```python
from build123d import *

# Parameters (mm, degrees)
F2_R     = 4.5
F3_DEPTH = 8
F4_W     = 30
F4_H     = 2
F5_DEPTH = 4.4


with BuildPart() as f1:
    # F0 (on Front) → F1 (revolve)
    with BuildSketch(Plane.XZ):
        Polygon((-7, 0), (0, 0), (0, 10), (-5, 10), (-5.25, 5.6), (-5, 5.6), (-5, 2), (-7, 2), align=None)
    revolve(axis=Axis((0, 0, 5), (0, 0, -1)))

    # F2 (on face) → F3 (cut)
    with BuildSketch(Plane.XY.offset(10)):
        Circle(F2_R)
    extrude(amount=-F3_DEPTH, mode=Mode.SUBTRACT)

    # F4 (on face) → F5 (cut)
    with BuildSketch(Plane.XY.offset(10)):
        with Locations((0.8593, 0)):
            Rectangle(F4_W, F4_H)
        with BuildLine():
            Line((-4.387482, 1), (4.387482, 1))
            ThreePointArc((4.387482, 1), (0, 4.5), (-4.387482, 1))
        make_face()
        with BuildLine():
            Line((15.8593, -1), (15.8593, 1))
            Line((15.8593, 1), (4.387482, 1))
            ThreePointArc((4.387482, 1), (4.471782, 0.503155), (4.5, 0))
            ThreePointArc((4.5, 0), (4.471782, -0.503155), (4.387482, -1))
            Line((4.387482, -1), (15.8593, -1))
        make_face()
    extrude(amount=-F5_DEPTH, mode=Mode.SUBTRACT)


solid = f1.part
```
Model file for the job. Use its own axes, mm. A direction names the side the tool comes from. Coordinates: 2 decimals unless noted, no trailing zeros. Loops run counter-clockwise (first coordinate to the right, second up) from the corner with the lowest first, then second, coordinate; pieces in that order, holes last. Notation, with made-up numbers: M -22,34.5 L -7,34.5 A16 ccw -7,63.5 Z; hole C -3,-40 d1. An arc over 180 degrees is marked long. Use CSV: the item, a comma, the result in double quotes. Start each with the question number.
1. Band-saw the part on D-D, the plane z = 4. List the corners of the cut face in (x, y), then the cut area to 3 significant figures.
2. Band-saw the part on B-B, the plane z = 7.75. List the corners of the cut face in (x, y).
3. Probe probe 1 along X at (y, z) = (0, 5.5); probe 2 along Y at (x, z) = (-3.25, 7.75). List the from-to ranges inside material, lowest first. Write a range as [from, to].
4. Band-saw the part on C-C, the plane y = 0. List the corners of the cut face in (x, z).
5. Two-plate mould, pull along Z, no slides. Class faces 1 (the cylindrical face through (-6.466, -2.681, 0.986)), 2 (the cylindrical face through (1.08, -4.88, 3.77)), 3 (the conical face through (-0.099, 5.126, 7.769)): pulls with the +Z half, pulls with the -Z half, needs draft (parallel to the pull), parting line crosses it, or undercut.
6. Tool access for faces 4 (the flat face through (0, 0, 2)), 5 (the conical face through (0.099, -5.126, 7.769)): list every direction of +Z, -Z, +X, -X, +Y, -Y with a clear straight run to the whole face (end or side of a thin tool).
7. Flat gauge pins, fed straight in: pin 1 (0.7 mm diameter, centred on x = -4.5, y = -0.5, fed in from +Z); pin 2 (0.8 mm diameter, centred on x = -4.5, z = 7, fed in from -Y); pin 3 (1.5 mm diameter, centred on x = -3, y = 5.5, fed in from +Z). Where does each tip first touch, or does it go through?
8. Band-saw the part on A-A, the plane x = 0. List the corners of the cut face in (y, z).
Entries:
1,outline,"C 0,0 d10; hole C 0,0 d9"
1,area,"14.9 mm2"
2,outline,"M -5.03,-1 A5.13 ccw 5.03,-1 L 4.39,-1 A4.5 cw -4.39,-1 Z; M -5.03,1 L -4.39,1 A4.5 cw 4.39,1 L 5.03,1 A5.13 ccw Z"
3,probe 1,"x = [-5, -4.5], [4.5, 5]"
3,probe 2,"y = [-3.97, -3.11], [3.11, 3.97]"
4,outline,"M -7,0 L 7,0 L 7,2 L 5,2 L 5,5.6 L 4.5,5.6 L 4.5,2 L -4.5,2 L -4.5,5.6 L -5,5.6 L -5,2 L -7,2 Z"
5,face 1,"needs draft"
5,face 2,"undercut"
5,face 3,"pulls with the +Z half"
6,face 4,"+Z"
6,face 5,"+Z, -Y"
7,pin 1,"stops at z = 5.6"
7,pin 2,"stops at y = -3.15"
7,pin 3,"stops at z = 2"
8,outline,"M -7,0 L 7,0 L 7,2 L 5,2 L 5,5.6 L 5.25,5.6 L 5,10 L 4.5,10 L 4.5,2 L -4.5,2 L -4.5,10 L -5,10 L -5.25,5.6 L -5,5.6 L -5,2 L -7,2 Z"
